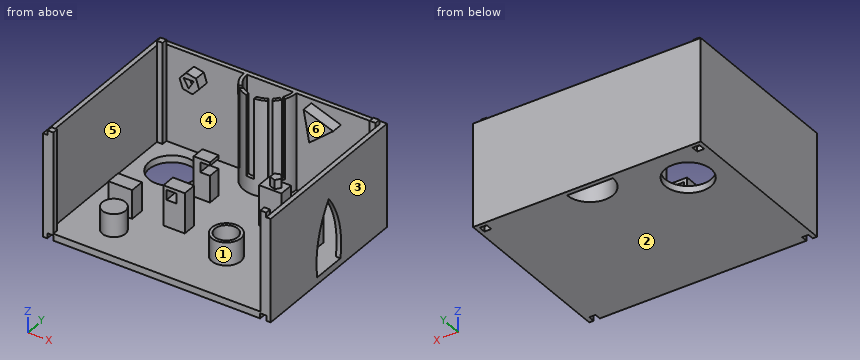
from build123d import *

# Parameters (mm, degrees)
F1_DEPTH  = 6
F2_DEPTH  = 90
F0_W      = 5
F0_H      = 5
F3_DEPTH  = 94
F4_W      = 5.5
F4_H      = 4.5
F5_DEPTH  = 5.5
F6_DEPTH  = 5.5
F7_R      = 20
F8_DEPTH  = 7
F9_DEPTH  = 6
F10_DEPTH = 84
F12_DEPTH = 4
F13_DEPTH = 5.5
F14_DEPTH = 25
F15_W     = 6
F15_H     = 6
F16_DEPTH = 4.5
F17_W     = 6
F17_H     = 6
F18_DEPTH = 4.5
F19_W     = 20.739749
F19_H     = 12.523103
F19_W_2   = 8.389108
F19_H_2   = 41.523981
F20_DEPTH = 25
F19_W_3   = 14.214885
F19_H_3   = 11.204887
F19_W_4   = 18.642471
F19_H_4   = 12.193553
F19_W_5   = 19.574596
F19_H_5   = 12.523113
F21_DEPTH = 35
F22_R     = 12.682536
F22_R_2   = 10.10667
F23_DEPTH = 20
F25_DEPTH = 10
F26_R     = 10
F27_DEPTH = 15
F28_W     = 8.713692
F28_H     = 8.713695
F29_DEPTH = 55
F31_DEPTH = 10
F33_DEPTH = 8
F35_DEPTH = 5
F37_DEPTH = 70


with BuildPart() as f1:
    # F0 (on Top) → F1 (new body)
    with BuildSketch(Plane.XY):
        Polygon((-90.5, -70), (-90.5, -75), (90.5, -75), (90.5, -70), (95.5, -70), (95.5, -66), (95.5, 66), (90.5, 66), (90.5, 71), (-90.5, 71), (-90.5, 66), (-95.5, 66), (-95.5, -66), (-95.5, -70), align=None)
        Polygon((99.5, 75), (-99.5, 75), (-99.5, -75), (-95.5, -75), (-95.5, -70), (-95.5, -66), (-95.5, 66), (-95.5, 71), (-90.5, 71), (90.5, 71), (95.5, 71), (95.5, 66), (95.5, -66), (95.5, -70), (95.5, -71), (95.5, -75), (99.5, -75), align=None)
    extrude(amount=F1_DEPTH)

    # F0 (on Top) → F2 (join)
    with BuildSketch(Plane.XY):
        Polygon((99.5, 75), (-99.5, 75), (-99.5, -75), (-95.5, -75), (-95.5, -70), (-95.5, -66), (-95.5, 66), (-95.5, 71), (-90.5, 71), (90.5, 71), (95.5, 71), (95.5, 66), (95.5, -66), (95.5, -70), (95.5, -71), (95.5, -75), (99.5, -75), align=None)
    extrude(amount=F2_DEPTH)

    # F0 (on Top) → F3 (join)
    with BuildSketch(Plane.XY):
        with Locations((-93, 68.5)):
            Rectangle(F0_W, F0_H)
        with Locations((93, 68.5)):
            Rectangle(F0_W, F0_H)
        Polygon((90.5, -75), (95.5, -75), (95.5, -71), (95.5, -70), (90.5, -70), align=None)
        with Locations((-93, -72.5)):
            Rectangle(F0_W, F0_H)
    extrude(amount=F3_DEPTH)

    # F4 (on face) → F5 (cut)
    with BuildSketch(Plane.XZ.offset(75)):
        with Locations((93, 2.25)):
            Rectangle(F4_W, F4_H)
    extrude(amount=-F5_DEPTH, mode=Mode.SUBTRACT)

    # F4 (on face) → F6 (cut)
    with BuildSketch(Plane.XZ.offset(75)):
        with Locations((-93, 2.25)):
            Rectangle(F4_W, F4_H)
    extrude(amount=F6_DEPTH, mode=Mode.SUBTRACT)

    # F7 (on face) → F8 (cut)
    with BuildSketch(Plane.XY.offset(6)):
        with Locations((-65.5, 41)):
            Circle(F7_R)
    extrude(amount=-F8_DEPTH, mode=Mode.SUBTRACT)

    # F7 (on face) → F9 (cut)
    with BuildSketch(Plane.XY.offset(6)):
        with BuildLine():
            Line((20, 71), (-20, 71))
            ThreePointArc((-20, 71), (0, 51), (20, 71))
        make_face()
    extrude(amount=-F9_DEPTH, mode=Mode.SUBTRACT)

    # F7 (on face) → F10 (join)
    with BuildSketch(Plane.XY.offset(6)):
        with BuildLine():
            Line((-20, 71), (-23, 71))
            ThreePointArc((-23, 71), (0, 48), (23, 71))
            Line((23, 71), (20, 71))
            ThreePointArc((20, 71), (0, 51), (-20, 71))
        make_face()
    extrude(amount=F10_DEPTH)

    # F11 (on face) → F12 (cut)
    with BuildSketch(Plane.YZ.offset(99.5)):
        with BuildLine():
            Line((-15.02791, 6), (14.97209, 6))
            ThreePointArc((14.97209, 6), (13.520819, 37.512182), (-0.02791, 66))
            ThreePointArc((-0.02791, 66), (-13.576638, 37.512182), (-15.02791, 6))
        make_face()
    extrude(amount=-F12_DEPTH, mode=Mode.SUBTRACT)

    # F4 (on face) → F13 (cut)
    with BuildSketch(Plane.XZ.offset(75)):
        with Locations((-93, 2.25)):
            Rectangle(F4_W, F4_H)
    extrude(amount=-F13_DEPTH, mode=Mode.SUBTRACT)

    # F0 (on Top) → F14 (join)
    with BuildSketch(Plane.XY):
        with Locations((-93, 68.5)):
            Rectangle(F0_W, F0_H)
    extrude(amount=F14_DEPTH)

    # F15 (on face) → F16 (cut)
    with BuildSketch(Plane(origin=(0, 0, 0), x_dir=(1, 0, 0), z_dir=(0, 0, -1))):
        with Locations((-93, -68.489519)):
            Rectangle(F15_W, F15_H)
    extrude(amount=-F16_DEPTH, mode=Mode.SUBTRACT)

    # F17 (on face) → F18 (cut)
    with BuildSketch(Plane(origin=(0, 0, 0), x_dir=(1, 0, 0), z_dir=(0, 0, -1))):
        with Locations((93, -68.5)):
            Rectangle(F17_W, F17_H)
    extrude(amount=-F18_DEPTH, mode=Mode.SUBTRACT)

    # F19 (on face) → F20 (join)
    with BuildSketch(Plane.XY.offset(6)):
        with Locations((-64.446979, -20.761568)):
            Rectangle(F19_W, F19_H)
        with Locations((73.623832, 4.284644)):
            Rectangle(F19_W_2, F19_H_2)
    extrude(amount=F20_DEPTH)

    # F19 (on face) → F21 (join)
    with BuildSketch(Plane.XY.offset(6)):
        with Locations((-26.462941, 27.683088)):
            Rectangle(F19_W_3, F19_H_3)
        with Locations((-21.219746, -15.323903)):
            Rectangle(F19_W_4, F19_H_4)
        with Locations((36.338889, 23.728418)):
            Rectangle(F19_W_5, F19_H_5)
    extrude(amount=F21_DEPTH)

    # F22 (on face) → F23 (join)
    with BuildSketch(Plane.XY.offset(6)):
        with Locations((29.347964, -28.670896)):
            Circle(F22_R)
        with Locations((-57.339538, -45.807783)):
            Circle(F22_R_2)
    extrude(amount=F23_DEPTH)

    # F24 (on face) → F25 (join)
    with BuildSketch(Plane.XZ.offset(-71)):
        Polygon((40.991751, 59.230904), (61.980041, 76.990236), (36.105864, 86.286962), align=None)
    extrude(amount=F25_DEPTH)

    # F26 (on face) → F27 (cut)
    with BuildSketch(Plane.XY.offset(26)):
        with Locations((29.347964, -28.670896)):
            Circle(F26_R)
    extrude(amount=-F27_DEPTH, mode=Mode.SUBTRACT)

    # F28 (on face) → F29 (cut)
    with BuildSketch(Plane.XZ.offset(21.42068)):
        with Locations((-23.41805, 33.660973)):
            Rectangle(F28_W, F28_H)
    extrude(amount=-F29_DEPTH, mode=Mode.SUBTRACT)

    # F30 (on face) → F31 (join)
    with BuildSketch(Plane.XZ.offset(-71)):
        Polygon((-60.947721, 63.067267), (-55.162239, 69.607382), (-57.933404, 77.887813), (-66.49005, 79.62813), (-72.275531, 73.088015), (-69.504367, 64.807584), align=None)
    extrude(amount=F31_DEPTH)

    # F32 (on face) → F33 (join)
    with BuildSketch(Plane.XY.offset(41)):
        Polygon((33.874482, 26.419034), (33.874482, 21.037802), (38.992337, 19.374911), (42.155346, 23.728418), (38.992337, 28.081926), align=None)
    extrude(amount=F33_DEPTH)

    # F34 (on face) → F35 (cut)
    with BuildSketch(Plane.XZ.offset(-61)):
        Polygon((-59.885368, 74.591823), (-68.859458, 74.591823), (-64.372413, 66.820033), align=None)
    extrude(amount=-F35_DEPTH, mode=Mode.SUBTRACT)

    # F36 (on face) → F37 (cut)
    with BuildSketch(Plane.XY.offset(90)):
        Polygon((1.664777, 54.871559), (-6.499225, 54.10137), (-4.958848, 46.553519), (1.664777, 46.553519), align=None)
        Polygon((11.985309, 56.951068), (9.674743, 54.640502), (12.293384, 49.865328), (15.402977, 51.570587), align=None)
        Polygon((-10.504208, 55.872802), (-13.81602, 58.183368), (-18.591192, 55.025596), (-16.126588, 53.177141), align=None)
        Polygon((16.837498, 61.957296), (16.307571, 59.421436), (20.30335, 57.413179), (21.556129, 59.905803), align=None)
    extrude(amount=-F37_DEPTH, mode=Mode.SUBTRACT)


solid = f1.part
Here's how the part is built. I have some questions about the finished solid (model axes, mm). Face numbers are marked on the shaded views. A direction names the side the tool comes from. Give positions to 0.01 mm unless a question says otherwise; leave off trailing zeros. Order: outer loops, then holes, each group sorted by start corner. A loop starts at its lowest first (then second) coordinate and runs counter-clockwise, first axis right, second up. Notation, with made-up numbers: (42.5, 24.25) -> (79.5, 24.25) arc R16 cw to (79.5, 53.25) -> close; hole circle Ø10 at (8, 75). An arc over 180 degrees is marked (long way). Use a Markdown table: item, result. Add a question column.
Item 1: If we mould it in two halves opening along X, with no side actions, what happens to the marked faces 1, 2 and 3? For each: pulls with the +X half, pulls with the -X half, needs draft (parallel to the pull), parting line crosses it, or undercut.
Item 2: Will these pins go through, and if not, where does the flat tip stop? pin 1 (3 mm diameter, centred on x = 93.5, y = 69, fed in from -Z); pin 2 (8 mm diameter, centred on x = -71, y = -45, fed in from +Z); pin 3 (2 mm diameter, centred on x = 24, y = 53, fed in from +Z).
Item 3: For the marked faces 4, 5 and 6, which set-ups out of +Z, -Z, +X, -X, +Y, -Y let a thin tool reach every point of the face, with its end or its side?
Item 4: I need wall thicknesses on line 1 (X direction, y = -53, z = 72); line 2 (Y direction, x = -65, z = 2); line 3 (X direction, y = 68, z = 49). Which ranges of each line are inside material? Lowest first, please.
Item 5: Imagine slicing it at C-C on y = 9.5. Please give me the cut outline in (x, z), plus the area to 3 significant figures.
Item 6: Imagine slicing it at B-B on x = -41. Please give me the cut outline in (y, z), plus the area to 3 significant figures.
Item 7: Imagine slicing it at A-A on y = 41. Please give me the cut outline in (x, z), plus the area to 3 significant figures.
Item 8: Imagine slicing it at D-D on z = 54.5. Give the number of separate pieces and of enclosed holes in the cut face, plus the area to 3 significant figures.
Data:
| question | item | result |
|---|---|---|
| 1 | face 1 | undercut |
| 1 | face 2 | needs draft |
| 1 | face 3 | pulls with the +X half |
| 2 | pin 1 | stops at z = 4.5 |
| 2 | pin 2 | stops at z = 26 |
| 2 | pin 3 | stops at z = 6 |
| 3 | face 4 | none |
| 3 | face 5 | +Z |
| 3 | face 6 | +Z, -Y |
| 4 | line 1 | x = -99.5 to -95.5, 95.5 to 99.5 |
| 4 | line 2 | y = -75 to 21.01, 60.99 to 75 |
| 4 | line 3 | x = -99.5 to -90.5, -22.8 to -19.77, 19.77 to 22.8, 90.5 to 99.5 |
| 5 | outline | (-99.5, 0) -> (99.5, 0) -> (99.5, 6) -> (77.82, 6) -> (77.82, 31) -> (69.43, 31) -> (69.43, 6) -> (-95.5, 6) -> (-95.5, 90) -> (-99.5, 90) -> close; (95.5, 49.48) -> (99.5, 49.48) -> (99.5, 90) -> (95.5, 90) -> close |
| 5 | area | 1,900 mm² |
| 6 | outline | (-75, 0) -> (75, 0) -> (75, 90) -> (71, 90) -> (71, 6) -> (-75, 6) -> close |
| 6 | area | 1,240 mm² |
| 7 | outline | (-99.5, 0) -> (-85.5, 0) -> (-85.5, 6) -> (-95.5, 6) -> (-95.5, 90) -> (-99.5, 90) -> close; (-45.5, 0) -> (99.5, 0) -> (99.5, 90) -> (95.5, 90) -> (95.5, 6) -> (-45.5, 6) -> close |
| 7 | area | 1,630 mm² |
| 8 | separate pieces | 5 |
| 8 | enclosed holes | 0 |
| 8 | area | 2,160 mm² |
